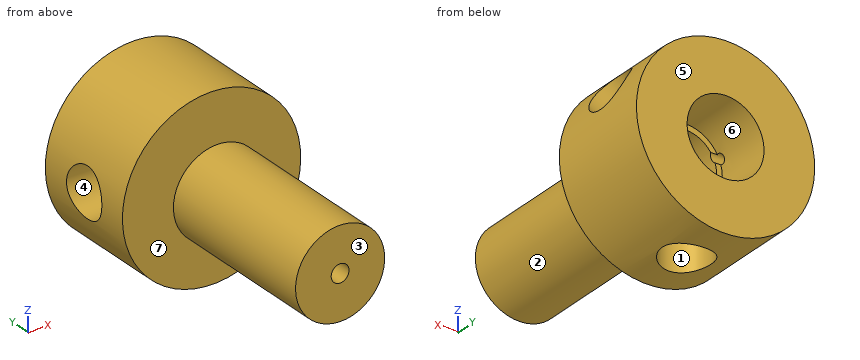
```python
from build123d import *

# Parameters (mm, degrees)
SKETCH1_R                    = 15.875
BOSS_EXTRUDE1_DEPTH          = 50.8
SKETCH2_OUTSIDE_W            = 47.31
SKETCH2_OUTSIDE_H            = 47.31
SKETCH2_OUTSIDE_R            = 7.9375
CUT_EXTRUDE1_DEPTH           = 31.75
F_1_8_0_125_DIAMETER_HOLE1_D = 3.175
CUT_EXTRUDE5_START           = -31.75
SKETCH13_OUTSIDE_W           = 47.31
SKETCH13_OUTSIDE_H           = 47.31
SKETCH13_OUTSIDE_R           = 6.35
CUT_EXTRUDE5_DEPTH           = 1.5875
CUT_EXTRUDE6_REACH           = 65.16
CUT_EXTRUDE6_END_RADIUS      = 15.875
CUT_EXTRUDE6_START           = -7.62
SKETCH15_R                   = 4.365625
CUT_EXTRUDE7_REACH           = 60.178
SKETCH16_R                   = 0.79375
CIRPATTERN1_COUNT            = 2
CIRPATTERN1_ANGLE            = 120
CIRPATTERN2_COUNT            = 2
CIRPATTERN2_ANGLE            = 270


with BuildPart() as part:
    # Sketch1 → Boss-Extrude1 (new body)
    with BuildSketch(Plane(origin=(0, 0, 0), x_dir=(1, 0, 0), z_dir=(0, 1, 0))):
        with Locations(Location((0, 0, 0), (0, 0, 270))):
            Circle(SKETCH1_R)
    extrude(amount=BOSS_EXTRUDE1_DEPTH)

    # Sketch2 outside → Cut-Extrude1 (cut)
    with BuildSketch(Plane(origin=(0, 0, 0), x_dir=(-1, 0, 0), z_dir=(0, -1, 0))):
        Rectangle(SKETCH2_OUTSIDE_W, SKETCH2_OUTSIDE_H)
        with Locations(Location((0, 0, 0), (0, 0, 90))):
            Circle(SKETCH2_OUTSIDE_R, mode=Mode.SUBTRACT)
    extrude(amount=-CUT_EXTRUDE1_DEPTH, mode=Mode.SUBTRACT)

    # 1/8 (0.125) Diameter Hole1 (through all)
    with Locations(Plane(origin=(0, 50.8, 0), x_dir=(1, 0, 0), z_dir=(0, 1, 0))):
        with Locations((0, 0)):
            Hole(F_1_8_0_125_DIAMETER_HOLE1_D / 2)

    # Sketch6 → 1/4 NPT Tapped Hole1 (revolve, cut)
    with BuildSketch(Plane(origin=(0, 50.8, 0), x_dir=(0, 0, 1), z_dir=(1, 0, 0))):
        Polygon((0, 0), (0, 20.275689079), (5.5626, 16.9333418), (5.5626, 9.906), (6.557984794, 9.906), (6.8545837, 0), align=None)
    revolve(axis=Axis((0, 57.15, 0), (0, -1, 0)), mode=Mode.SUBTRACT)

    # Sketch13 outside → Cut-Extrude5 (cut)
    with BuildSketch(Plane.XZ.offset(CUT_EXTRUDE5_START)):
        Rectangle(SKETCH13_OUTSIDE_W, SKETCH13_OUTSIDE_H)
        with Locations(Location((0, 0, 0), (0, 0, 270))):
            Circle(SKETCH13_OUTSIDE_R, mode=Mode.SUBTRACT)
    extrude(amount=CUT_EXTRUDE5_DEPTH, mode=Mode.SUBTRACT)

    # Cut-Extrude6: up to this cylinder (the profile starts inside it)
    cut_extrude6_end = Plane(origin=(0, 41.207118, 0), z_dir=(0, -1, 0)) * Cylinder(CUT_EXTRUDE6_END_RADIUS, 163.07, mode=Mode.PRIVATE)
    # Sketch15 → Cut-Extrude6 (cut, up to the surface)
    with BuildSketch(Plane.XY.offset(CUT_EXTRUDE6_START), mode=Mode.PRIVATE) as cut_extrude6_sk1:
        with Locations((0, 41.207117901)):
            Circle(SKETCH15_R)
    cut_extrude6_tool1 = extrude(cut_extrude6_sk1.sketch, amount=-CUT_EXTRUDE6_REACH, mode=Mode.PRIVATE) & cut_extrude6_end
    cut_extrude6 = cut_extrude6_tool1.solids().sort_by_distance((0, 41.207118, -7.62))[0]
    add(cut_extrude6, mode=Mode.SUBTRACT)

    # Sketch16 → Cut-Extrude7 (cut, up to next)
    with BuildSketch(Plane(origin=(0, 0, -7.62), x_dir=(-1, 0, 0), z_dir=(0, 0, -1)), mode=Mode.PRIVATE) as cut_extrude7_sk1:
        with Locations((2.54, 41.207117901)):
            Circle(SKETCH16_R)
    cut_extrude7_tool1 = extrude(cut_extrude7_sk1.sketch, amount=-CUT_EXTRUDE7_REACH, mode=Mode.PRIVATE) & part.part
    cut_extrude7 = cut_extrude7_tool1.solids().sort_by_distance((-2.54, 41.207118, -7.62))[0]
    add(cut_extrude7, mode=Mode.SUBTRACT)

    # CirPattern1: Cut-Extrude6, Cut-Extrude7 ×2 about axis
    cirpattern1_axis = Axis((0, 50.8, 0), (0, -1, 0))
    add([cut_extrude6.rotate(cirpattern1_axis, i * CIRPATTERN1_ANGLE / (CIRPATTERN1_COUNT - 1)) for i in range(1, CIRPATTERN1_COUNT)], mode=Mode.SUBTRACT)
    add([cut_extrude7.rotate(cirpattern1_axis, i * CIRPATTERN1_ANGLE / (CIRPATTERN1_COUNT - 1)) for i in range(1, CIRPATTERN1_COUNT)], mode=Mode.SUBTRACT)

    # CirPattern2: Cut-Extrude6, Cut-Extrude7 ×2 about axis
    cirpattern2_axis = Axis((0, 50.8, 0), (0, -1, 0))
    add([cut_extrude6.rotate(cirpattern2_axis, i * CIRPATTERN2_ANGLE / (CIRPATTERN2_COUNT - 1)) for i in range(1, CIRPATTERN2_COUNT)], mode=Mode.SUBTRACT)
    add([cut_extrude7.rotate(cirpattern2_axis, i * CIRPATTERN2_ANGLE / (CIRPATTERN2_COUNT - 1)) for i in range(1, CIRPATTERN2_COUNT)], mode=Mode.SUBTRACT)


solid = part.part
```
Work out the finished part from the listing and answer in its coordinate system (mm). Face numbers are marked on the shaded views. A direction names the side the tool comes from. Give positions to 0.01 mm unless a question says otherwise; leave off trailing zeros. Order: outer loops, then holes, each group sorted by start corner. A loop starts at its lowest first (then second) coordinate and runs counter-clockwise, first axis right, second up.
1. Straight lines are drawn through the part: L1, parallel to Y at x = -2, z = 7.5; L2, parallel to Z at x = 0, y = 39.25 (3 decimals); L3, parallel to Y at x = -14, z = 0. For each, find the intervals that lie inside material, in ascending order.
Result sheet:
L1: y = 0 to 30.16, 31.75 to 50.8
L2: z = -7.62 to -5.563, 5.563 to 15.875
L3: y = 31.75 to 36.84, 45.57 to 50.8
2. Each of these flat-tipped pins is pushed along its axis until it touches: P1, Ø2, axis at y = 11, z = -3.5, coming from the -X side; P2, Ø2, axis at x = 1.5, z = -3, coming from the +Y side; P3, Ø6, axis at y = 42, z = -6.5, coming from the -X side; P4, Ø1.9, axis at x = 0, z = 0, coming from the -Y side. Where does it stop, or does it pass through?
Result sheet:
P1: stops at x = -7.53
P2: stops at y = 33.14
P3: stops at x = -15.41
P4: passes through
3. Section B-B, the plane y = 21 is taken. Determine the outline of the cut face in (x, z) (1 decimal), and give its area (3 significant figures).
Result sheet:
outline: circle Ø15.9 at (0, 0); hole circle Ø3.2 at (0, 0)
area: 190 mm2
4. Section D-D, the plane y = 47 is taken. Determine the outline of the cut face in (x, z) (3 decimals).
Result sheet:
outline: circle Ø31.75 at (0, 0); hole circle Ø13.482 at (0, 0)
5. For the marked faces 4, 5, 6 and 7, determine the directions among +Z, -Z, +X, -X, +Y, -Y from which every point of the face is accessible in a straight line to the end or side of a thin tool.
Result sheet:
face 4: -X
face 5: +Z, -Z, +X, -X, +Y
face 6: +Y
face 7: none
6. Section C-C, the plane z = -10.5 is taken. Determine the outline of the cut face in (x, y).
Result sheet:
outline: (-11.91, 31.75) - (11.91, 31.75) - (11.91, 50.8) - (-11.91, 50.8) - close; hole circle Ø8.73 at (0, 41.21)
7. The mould has two halves that part along X. Classify the marked faces 1, 2 and 3: released by +X, released by -X, zero draft, split by the parting line, or undercut.
Result sheet:
face 1: undercut
face 2: split by the parting line
face 3: zero draft
